Design review of the part shown in the three views and the two pictorial views. Dimensions are in mm from the part's minimum x, y and z. A direction names the side the tool comes from. Give positions to 0.01 mm unless a question says otherwise; leave off trailing zeros. Loops run counter-clockwise (first coordinate to the right, second up) from the corner with the lowest first, then second, coordinate; pieces in that order, holes last. Notation, with made-up numbers: (35.25, -26) - (56.25, -26) arc R12 cw to (56.25, -15) - close; hole circle Ø10 at (68, 4). An arc over 180 degrees is marked (long way). Use CSV: the item, a comma, the result in double quotes. Start each with the question number.
1. Take a section at C-C on y = 1.5. Give the boundary of the cut face in (x, z).
2. Take a section at A-A on x = 26. Give the boundary of the cut face in (y, z).
3. Wall thickness on line 1 (Z direction, x = 28.5, y = 4); line 2 (Y direction, x = 16, z = 25.5): over which ranges is each line inside the solid? List them lowest first.
4. For pin 1 (5 mm diameter, centred on y = 4, z = 8.5, fed in from +X); pin 2 (6 mm diameter, centred on y = 15.5, z = 14.5, fed in from +X); pin 3 (6 mm diameter, centred on y = 3.5, z = 6, fed in from +X), all flat-tipped, find the tip position at first contact; note any pin that passes through.
5. For the marked faces 1 and 2, list the 3-axis set-ups (+Z, -Z, +X, -X, +Y, -Y) from which the entire face can be reached by the end or side of a thin tool; tool diameter is ignored.
6. Take a section at B-B on z = 27. Give the boundary of the cut face in (x, y), plus the area to 3 significant figures.
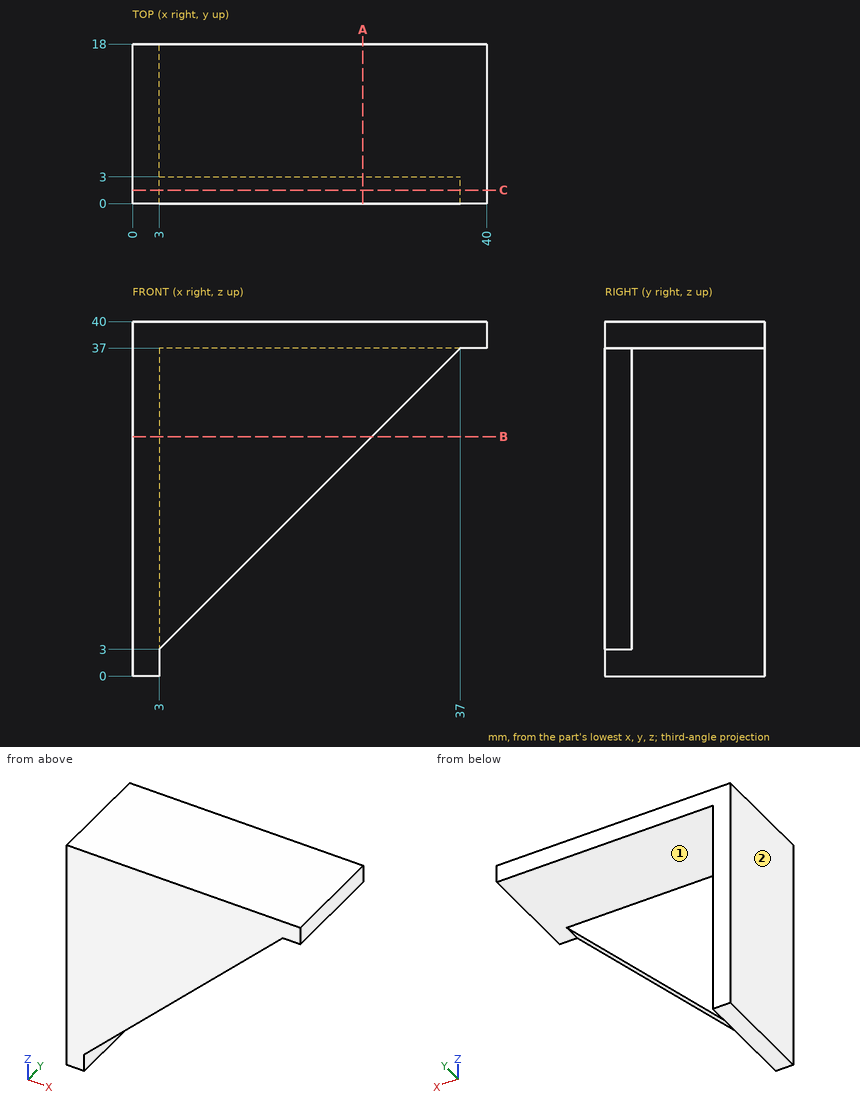
Check result:
1,outline,"(0, 0) - (3, 0) - (3, 3) - (37, 37) - (40, 37) - (40, 40) - (0, 40) - close"
2,outline,"(0, 26) - (3, 26) - (3, 37) - (18, 37) - (18, 40) - (0, 40) - close"
3,line 1,"z = 37 to 40"
3,line 2,"y = 0 to 3"
4,pin 1,"stops at x = 10.79"
4,pin 2,"stops at x = 3"
4,pin 3,"stops at x = 8.96"
5,face 1,"-Z, +X, +Y"
5,face 2,"+Z, -Z, -X, +Y, -Y"
6,outline,"(0, 0) - (27, 0) - (27, 3) - (3, 3) - (3, 18) - (0, 18) - close"
6,area,"126 mm²"
